The model under review builds one solid part; all positions refer to its coordinate system, in mm. A direction names the side the tool comes from. Round coordinates to 2 decimals unless told otherwise and drop trailing zeros. Write each loop counter-clockwise with the first axis right and the second up, starting at its lowest first coordinate (ties: lowest second). Pieces come first, ordered by that corner, then holes. Notation, with made-up numbers: (-23.75, 4) -> (8.25, 4) arc R27 ccw to (8.25, 43) -> close; hole circle Ø8 at (80.5, 22). An arc over 180 degrees is marked (long way). Use CSV: the item, a comma, the result in double quotes. Start each with the question number.
1) Take a section at A-A, the plane z = -0.25. Give the boundary of the cut face in (x, y), then the cut area to 3 significant figures.
2) For pin 1 Ø3 at (y, z) = (7, 4) entering from +X; pin 2 Ø1 at (y, z) = (-1, 2) entering from +X; pin 3 Ø1.5 at (x, z) = (75, 6.5) entering from -Y; pin 4 Ø3 at (x, z) = (67.5, 4.5) entering from +Y, all flat-tipped, find the tip position at first contact; note any pin that passes through.
3) Mouldability with a two-part tool opening along Z and no side actions: class faces 3 (the face through (73, 11, 0)), 4 (the face through (73, 0, 7)), 5 (the face through (68.255, 6.142, 3.437)), 6 (the face through (70, 8, -1)) as released by +Z, released by -Z, zero draft, split by the parting line, or undercut.
4) Wall thickness on probe 1 along Z at (x, y) = (66.5, -1); probe 2 along Y at (x, z) = (69.25, 5.5); probe 3 along Y at (x, z) = (71, 1.25): over which ranges is each line inside the solid? List them lowest first. Write a range as [from, to].
5) Machinability: for faces 1 (the face through (75.274, 3.374, 3.451)), 2 (the face through (78.27, 2.99, -0.65)), which of the approach directions +Z, -Z, +X, -X, +Y, -Y give a long, thin tool a straight path to every point of the face, cutting with its end or side? Answer none if there is none.
6) Take a section at B-B, the plane z = 2.75. Give the boundary of the cut face in (x, y), then the cut area to 3 significant figures.
from build123d import *

# Parameters (mm, degrees)
SKETCH1_R           = 6.05
BOSS_EXTRUDE1_DEPTH = 7
SKETCH4_R           = 9
BOSS_EXTRUDE2_DEPTH = 1
BOSS_EXTRUDE3_START = 1
SKETCH6_R           = 9
BOSS_EXTRUDE3_DEPTH = 1
FILLET1_R           = 0.5
FILLET2_R           = 0.5
FILLET3_R           = 0.2
FILLET4_R           = 0.2
SKETCH11_R          = 1.5
CUT_EXTRUDE1_DEPTH  = 81.5497711


with BuildPart() as part:
    # Sketch1 → Boss-Extrude1 (new body)
    with BuildSketch(Plane.XY):
        with Locations((69.685635463, 5.691370847)):
            Circle(SKETCH1_R)
    extrude(amount=BOSS_EXTRUDE1_DEPTH)

    # Sketch4 → Boss-Extrude2 (add)
    with BuildSketch(Plane.XY.offset(7)):
        with Locations((69.685635463, 5.691370847)):
            Circle(SKETCH4_R)
    extrude(amount=BOSS_EXTRUDE2_DEPTH)

    # Sketch6 → Boss-Extrude3 (add)
    with BuildSketch(Plane(origin=(0, 0, 0), x_dir=(-1, 0, 0), z_dir=(0, 0, -1)).offset(BOSS_EXTRUDE3_START)):
        with Locations(Location((-69.685635463, 5.691370847, 0), (0, 0, 180))):
            Circle(SKETCH6_R)
    extrude(amount=-BOSS_EXTRUDE3_DEPTH)

    # Fillet1
    fillet1_edges = [part.edges().sort_by_distance(p)[0] for p in [
        (60.685635463, 5.691370847, 0),
    ]]
    fillet(fillet1_edges, radius=FILLET1_R)

    # Fillet2
    fillet2_edges = [part.edges().sort_by_distance(p)[0] for p in [
        (60.685635463, 5.691370847, 7),
    ]]
    fillet(fillet2_edges, radius=FILLET2_R)

    # Fillet3
    fillet3_edges = [part.edges().sort_by_distance(p)[0] for p in [
        (60.685635463, 5.691370847, 8),
    ]]
    fillet(fillet3_edges, radius=FILLET3_R)

    # Fillet4
    fillet4_edges = [part.edges().sort_by_distance(p)[0] for p in [
        (60.685635463, 5.691370847, -1),
    ]]
    fillet(fillet4_edges, radius=FILLET4_R)

    # Sketch11 → Cut-Extrude1 (cut, through all)
    with BuildSketch(Plane(origin=(0, 0, -1), x_dir=(-1, 0, 0), z_dir=(0, 0, -1))):
        with Locations((-69.685635463, 5.691370847)):
            Circle(SKETCH11_R)
    extrude(amount=-CUT_EXTRUDE1_DEPTH, mode=Mode.SUBTRACT)


solid = part.part
Values found:
1,outline,"circle Ø17.87 at (69.69, 5.69); hole circle Ø3 at (69.69, 5.69)"
1,area,"244 mm²"
2,pin 1,"x = 75.74"
2,pin 2,"through"
2,pin 3,"y = -1.66"
2,pin 4,"y = 11.7"
3,face 3,"undercut"
3,face 4,"undercut"
3,face 5,"zero draft"
3,face 6,"released by -Z"
4,probe 1,"[-1, 0], [7, 8]"
4,probe 2,"[-0.34, 4.26], [7.13, 11.73]"
4,probe 3,"[-0.21, 4.97], [6.41, 11.6]"
5,face 1,"none"
5,face 2,"+Z, -Z"
6,outline,"circle Ø12.1 at (69.69, 5.69); hole circle Ø3 at (69.69, 5.69)"
6,area,"108 mm²"
